Read the model definition and answer for the solid it produces. Units are mm, in the model's axes. Face numbers are marked on the shaded views. A direction names the side the tool comes from. Round coordinates to 2 decimals unless told otherwise and drop trailing zeros. Order: outer loops, then holes, each group sorted by start corner. A loop starts at its lowest first (then second) coordinate and runs counter-clockwise, first axis right, second up. Notation, with made-up numbers: (35, 19.5) -> (83, 19.5) arc R19 ccw to (83, 54.5) -> close; hole circle Ø9 at (-34.75, -24.5). An arc over 180 degrees is marked (long way). Answer as a JSON object with one key per item and string values. Group by question number.
Item 1: Given P1, Ø0.6, axis at x = 1.5, z = 0, coming from the +Y side; P2, Ø1.1, axis at x = 0, z = -1, coming from the +Y side, each flat-ended and moving along its own axis, determine where each tip first touches the part or whether it passes through.
Item 2: The mould has two halves that part along Z. Classify the marked faces 4, 5 and 6: pulls with the +Z half, pulls with the -Z half, needs draft (parallel to the pull), parting line crosses it, or undercut.
Item 3: Section C-C, the plane z = 0 is taken. Write down the section's boundary in (x, y) (3 decimals).
Item 4: Section A-A, the plane y = 4.5 is taken. Write down the section's boundary in (x, z) (3 decimals), plus the area to 3 significant figures.
Item 5: Section D-D, the plane y = 1 is taken. Write down the section's boundary in (x, z), plus the area to 3 significant figures.
Item 6: For the marked faces 1, 2 and 3, determine the directions among +Z, -Z, +X, -X, +Y, -Y from which every point of the face is accessible in a straight line to the end or side of a thin tool.
Item 7: Consider probe 1 along Z at (x, y) = (1.25, 2.75); probe 2 along X at (y, z) = (5.25, 0.7); probe 3 along Z at (x, y) = (0.75, 5). Determine where each line is inside the solid, lowest interval first. Write a range as from..to.
Item 8: Section B-B, the plane x = 1.26 is taken. Write down the section's boundary in (y, z) (3 decimals).
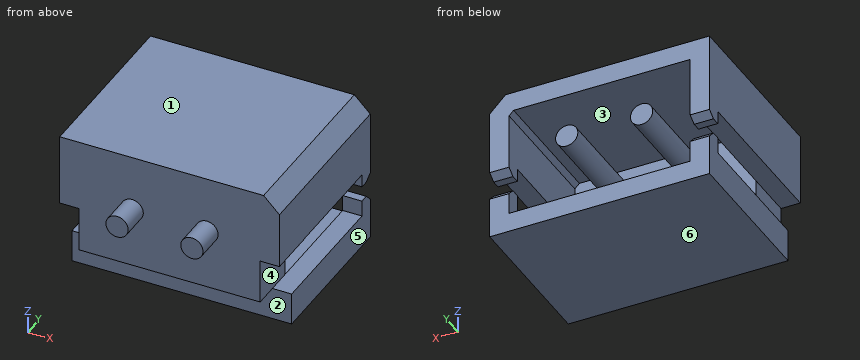
from build123d import *

# Parameters (mm, degrees)
SKETCH1_R                  = 0.375
BOSS_EXTRUDE1_DEPTH        = 5.7
BOSS_EXTRUDE1_DEPTH_BACK   = 1
BOSS_EXTRUDE1_2_DEPTH      = 5.7
BOSS_EXTRUDE1_2_DEPTH_BACK = 1
BOSS_EXTRUDE2_DEPTH        = 1.65
BOSS_EXTRUDE4_DEPTH        = 6
SKETCH5_W                  = 8.470715742
SKETCH5_H                  = 1.5
CUT_EXTRUDE1_DEPTH         = 4.35
BOSS_EXTRUDE5_DEPTH        = 0.65
BOSS_EXTRUDE6_DEPTH        = 0.65
SKETCH8_W                  = 1.741902436
SKETCH8_H                  = 1.335943606
CUT_EXTRUDE2_DEPTH         = 4.7
CUT_EXTRUDE2_DEPTH_BACK    = 4.7
SKETCH10_W                 = 0.65
SKETCH10_H                 = 1.488696467
SKETCH10_H_2               = 1.5
CUT_EXTRUDE3_DEPTH         = 10


with BuildPart() as part:
    # Sketch1 → Boss-Extrude1 (new body, two sides)
    with BuildSketch(Plane(origin=(0, 0, 0), x_dir=(1, 0, 0), z_dir=(0, 1, 0))) as boss_extrude1_sk:
        with Locations((-1.26, 0)):
            Circle(SKETCH1_R)
    extrude(amount=BOSS_EXTRUDE1_DEPTH)
    extrude(boss_extrude1_sk.sketch, amount=-BOSS_EXTRUDE1_DEPTH_BACK)



with BuildPart() as body_2:
    # Sketch1 → Boss-Extrude1 2 (new body, two sides)
    with BuildSketch(Plane(origin=(0, 0, 0), x_dir=(1, 0, 0), z_dir=(0, 1, 0))) as boss_extrude1_2_sk:
        with Locations((1.26, 0)):
            Circle(SKETCH1_R)
    extrude(amount=BOSS_EXTRUDE1_2_DEPTH)
    extrude(boss_extrude1_2_sk.sketch, amount=-BOSS_EXTRUDE1_2_DEPTH_BACK)


with BuildPart() as part_1:
    add(part.part)

    add(body_2.part)  # Boss-Extrude2 merges body 2
    # Sketch2 → Boss-Extrude2 (add)
    with BuildSketch(Plane(origin=(0, 0, 0), x_dir=(1, 0, 0), z_dir=(0, 1, 0))):
        Polygon((3.7, -1.365567335), (3.165567335, -1.9), (-3.7, -1.9), (-3.7, 3.1), (3.7, 3.1), align=None)
    extrude(amount=BOSS_EXTRUDE2_DEPTH)

    # Sketch4 → Boss-Extrude4 (add)
    with BuildSketch(Plane(origin=(0, 0, 0), x_dir=(1, 0, 0), z_dir=(0, 1, 0))):
        Polygon((3.165567335, -1.9), (3.7, -1.365567335), (3.7, 3.1), (-3.7, 3.1), (-3.7, -1.9), align=None)
        Polygon((-3.05, -1.25), (2.89632852, -1.25), (3.05, -1.09632852), (3.05, 2.45), (-3.05, 2.45), align=None, mode=Mode.SUBTRACT)
    extrude(amount=BOSS_EXTRUDE4_DEPTH)

    # Sketch5 → Cut-Extrude1 (cut)
    with BuildSketch(Plane(origin=(0, 6, 0), x_dir=(1, 0, 0), z_dir=(0, 1, 0))):
        with Locations((0, 1.259795506)):
            Rectangle(SKETCH5_W, SKETCH5_H)
    extrude(amount=-CUT_EXTRUDE1_DEPTH, mode=Mode.SUBTRACT)

    # Sketch6 → Boss-Extrude5 (add)
    with BuildSketch(Plane.ZY.offset(3.7)):
        Polygon((-2.009795506, 6), (-1.731148103, 6), (-1.467778214, 5.736630111), (-1.467778214, 5.451734295), (-2.009795506, 5.451734295), align=None)
        Polygon((-0.509795506, 6), (-0.768050416, 6), (-0.950007845, 5.736630111), (-0.950007845, 5.451734295), (-0.509795506, 5.451734295), align=None)
    extrude(amount=-BOSS_EXTRUDE5_DEPTH)

    # Sketch7 → Boss-Extrude6 (add)
    with BuildSketch(Plane(origin=(3.7, 0, 0), x_dir=(0, 0, -1), z_dir=(1, 0, 0))):
        Polygon((0.768050416, 6), (0.509795506, 6), (0.509795506, 5.451734295), (0.950007845, 5.451734295), (0.950007845, 5.736630111), align=None)
        Polygon((2.009795506, 6), (1.731148103, 6), (1.467778214, 5.736630111), (1.467778214, 5.451734295), (2.009795506, 5.451734295), align=None)
    extrude(amount=-BOSS_EXTRUDE6_DEPTH)

    # Sketch8 → Cut-Extrude2 (cut, two sides)
    with BuildSketch(Plane(origin=(0, 0, 0), x_dir=(0, 0, -1), z_dir=(1, 0, 0))) as cut_extrude2_sk:
        with Locations((2.880746724, 0.138578557)):
            Rectangle(SKETCH8_W, SKETCH8_H)
    extrude(amount=CUT_EXTRUDE2_DEPTH, mode=Mode.SUBTRACT)
    extrude(cut_extrude2_sk.sketch, amount=-CUT_EXTRUDE2_DEPTH_BACK, mode=Mode.SUBTRACT)

    # Sketch10 → Cut-Extrude3 (cut)
    with BuildSketch(Plane(origin=(0, 1.65, 0), x_dir=(1, 0, 0), z_dir=(0, 1, 0))):
        with Locations((3.375, 1.265447273)):
            Rectangle(SKETCH10_W, SKETCH10_H)
        with Locations((-3.375, 1.259795506)):
            Rectangle(SKETCH10_W, SKETCH10_H_2)
    extrude(amount=-CUT_EXTRUDE3_DEPTH, mode=Mode.SUBTRACT)


solid = part_1.part
Values found:
{
 "1": {"P1": "y = 5.7", "P2": "y = 1.65"},
 "2": {"face 4": "undercut", "face 5": "needs draft", "face 6": "pulls with the -Z half"},
 "3": {"outline": "(-3.7, 0) -> (-1.635, 0) -> (-1.635, -1) -> (-0.885, -1) -> (-0.885, 0) -> (0.885, 0) -> (0.885, -1) -> (1.635, -1) -> (1.635, 0) -> (3.7, 0) -> (3.7, 6) -> (3.05, 6) -> (3.05, 1.65) -> (1.635, 1.65) -> (1.635, 5.7) -> (0.885, 5.7) -> (0.885, 1.65) -> (-0.885, 1.65) -> (-0.885, 5.7) -> (-1.635, 5.7) -> (-1.635, 1.65) -> (-3.05, 1.65) -> (-3.05, 6) -> (-3.7, 6) -> close"},
 "4": {"outline": "(-3.7, -3.1) -> (3.7, -3.1) -> (3.7, -2.01) -> (3.05, -2.01) -> (3.05, -2.45) -> (-3.05, -2.45) -> (-3.05, -2.01) -> (-3.7, -2.01) -> close; (-3.7, -0.51) -> (-3.05, -0.51) -> (-3.05, 1.25) -> (2.896, 1.25) -> (3.05, 1.096) -> (3.05, -0.51) -> (3.7, -0.51) -> (3.7, 1.366) -> (3.166, 1.9) -> (-3.7, 1.9) -> close; circle Ø0.75 at (-1.26, 0); circle Ø0.75 at (1.26, 0)", "area": "13.2 mm2"},
 "5": {"outline": "(-3.7, -3.1) -> (3.7, -3.1) -> (3.7, -2.01) -> (3.05, -2.01) -> (3.05, -0.52) -> (3.7, -0.52) -> (3.7, 1.37) -> (3.17, 1.9) -> (-3.7, 1.9) -> (-3.7, -0.51) -> (-3.05, -0.51) -> (-3.05, -2.01) -> (-3.7, -2.01) -> close", "area": "34.9 mm2"},
 "6": {"face 1": "+Z, +X, -X, +Y, -Y", "face 2": "-Z, +X, -X, -Y", "face 3": "+Y"},
 "7": {"probe 1": "-3.1..-2.45, -0.37..0.37, 1.25..1.9", "probe 2": "-3.7..-3.05, 3.05..3.7", "probe 3": "-3.1..-2.45, 1.25..1.9"},
 "8": {"outline": "(-1, -0.375) -> (0, -0.375) -> (0, -2.01) -> (0.807, -2.01) -> (0.807, -3.1) -> (6, -3.1) -> (6, -2.45) -> (1.65, -2.45) -> (1.65, -0.375) -> (5.7, -0.375) -> (5.7, 0.375) -> (1.65, 0.375) -> (1.65, 1.25) -> (6, 1.25) -> (6, 1.9) -> (0, 1.9) -> (0, 0.375) -> (-1, 0.375) -> close"}
}
